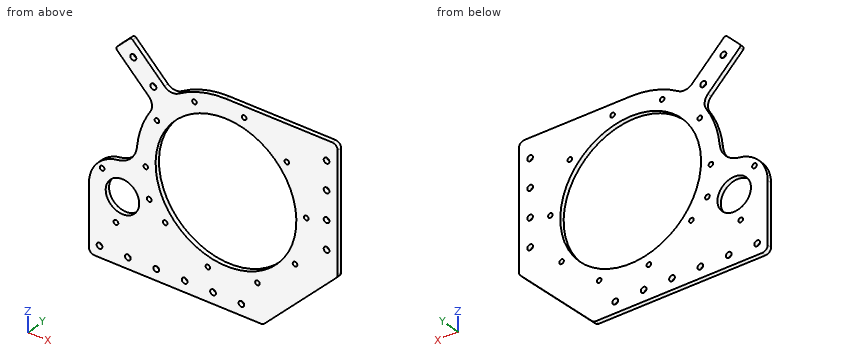
```python
from build123d import *

# Parameters (mm, degrees)
SKETCH_1_R               = 80
SKETCH_1_R_2             = 63
EXTRUDE_1_DEPTH          = 4
EXTRUDE_START            = -4
EXTRUDE_2_DEPTH          = 4
SKETCH_3_R               = 2.1
CUT_EXTRUDE_1_DEPTH      = 10
SKETCH_4_R               = 2.05
CUT_EXTRUDE_2_DEPTH      = 10
PATTERN_CIRCULAR_1_COUNT = 10
SKETCH_5_W               = 20
SKETCH_5_H               = 113.13708499
SKETCH_5_W_2             = 155.80242317
SKETCH_5_H_2             = 20
EXTRUDE_3_DEPTH          = 4
SKETCH_6_R               = 2.55
CUT_EXTRUDE_3_DEPTH      = 10
FILLET_1_R               = 20
SKETCH_7_R               = 15
CUT_EXTRUDE_4_DEPTH      = 10
FILLET_2_R               = 5
SKETCH_8_W               = 256.678769512
SKETCH_8_H               = 176.797047192
CUT_EXTRUDE_5_DEPTH      = 290
EXTRUDE_4_DEPTH          = 4
FILLET_3_R               = 10
FILLET_4_R               = 2
CUT_EXTRUDE_6_DEPTH      = 10


with BuildPart() as part:
    # 草图1 → 凸台-拉伸1 (new body)
    # profile 1 of 5: a face of its own
    with BuildSketch(Plane(origin=(0, 0, 0), x_dir=(1, 0, 0), z_dir=(0, 1, 0))):
        with BuildLine():
            ThreePointArc((0, -80), (-56.568542608, -56.568542382), (-80, 3.2e-07))
            Line((-80, 3.2e-07), (-80, -80))
            Line((-80, -80), (0, -80))
        make_face()
    # profile 2 of 5: a face of its own
    with BuildSketch(Plane(origin=(0, 0, 0), x_dir=(1, 0, 0), z_dir=(0, 1, 0))):
        Circle(SKETCH_1_R)
        with Locations(Location((0, 0, 0), (0, 0, 270))):
            Circle(SKETCH_1_R_2, mode=Mode.SUBTRACT)
    # profile 3 of 5: a face of its own
    with BuildSketch(Plane(origin=(0, 0, 0), x_dir=(1, 0, 0), z_dir=(0, 1, 0))):
        with BuildLine():
            ThreePointArc((-80, 3.2e-07), (-73.91036254, 30.614674737), (-56.568542495, 56.568542495))
            Line((-56.568542495, 56.568542495), (-80, 33.13708499))
            Line((-80, 33.13708499), (-80, 3.2e-07))
        make_face()
    # profile 4 of 5: a face of its own
    with BuildSketch(Plane(origin=(0, 0, 0), x_dir=(1, 0, 0), z_dir=(0, 1, 0))):
        with BuildLine():
            Line((0, 80), (-33.13708499, 80))
            Line((-33.13708499, 80), (-56.568542495, 56.568542495))
            ThreePointArc((-56.568542495, 56.568542495), (-30.614674589, 73.910362601), (0, 80))
        make_face()
    # profile 5 of 5: a face of its own
    with BuildSketch(Plane(origin=(0, 0, 0), x_dir=(1, 0, 0), z_dir=(0, 1, 0))):
        with BuildLine():
            Line((80, 80), (0, 80))
            ThreePointArc((0, 80), (56.568542495, 56.568542495), (80, 0))
            Line((80, 0), (80, 80))
        make_face()
    extrude(amount=EXTRUDE_1_DEPTH)


with BuildPart() as body_2:
    # 草图2 → 凸台-拉伸2 (new body)
    with BuildSketch(Plane(origin=(0, 4, 0), x_dir=(1, 0, 0), z_dir=(0, 1, 0)).offset(EXTRUDE_START)):
        with BuildLine():
            Line((122.66533818, 80), (80, 80))
            Line((80, 80), (80, 10))
            Line((80, 10), (92.66533818, 10))
            ThreePointArc((92.66533818, 10), (113.878541616, 18.786796564), (122.66533818, 40))
            Line((122.66533818, 40), (122.66533818, 80))
        make_face()
    extrude(amount=EXTRUDE_2_DEPTH)


with BuildPart() as part_1:
    add(part.part)

    # Combine 5: union body 2
    add(body_2.part)

    # 草图3 → 切除-拉伸1 (cut)
    with BuildSketch(Plane(origin=(0, 4, 0), x_dir=(1, 0, 0), z_dir=(0, 1, 0))):
        with Locations(Location((98.488743184, 64.31230047, 0), (0, 0, 270))):
            Circle(SKETCH_3_R)
        with Locations(Location((110.808705509, 22.800633094, 0), (0, 0, 270))):
            Circle(SKETCH_3_R)
        with Locations(Location((68.698565846, 32.887066435, 0), (0, 0, 270))):
            Circle(SKETCH_3_R)
    extrude(amount=-CUT_EXTRUDE_1_DEPTH, mode=Mode.SUBTRACT)

    # 草图4 → 切除-拉伸2 (cut)
    with BuildSketch(Plane(origin=(0, 4, 0), x_dir=(1, 0, 0), z_dir=(0, 1, 0))):
        with Locations(Location((-71.825637732, -6.283929052, 0), (0, 0, 270))):
            Circle(SKETCH_4_R)
    cut_extrude_2 = extrude(amount=-CUT_EXTRUDE_2_DEPTH, mode=Mode.SUBTRACT)

    # 阵列(圆周)1: 切除-拉伸2 ×10 about axis
    pattern_circular_1_axis = Axis((0, 0, 0), (0, 1, 0))
    for i in range(1, PATTERN_CIRCULAR_1_COUNT):
        add(cut_extrude_2.rotate(pattern_circular_1_axis, i * 360 / PATTERN_CIRCULAR_1_COUNT), mode=Mode.SUBTRACT)

    # 草图5 → 凸台-拉伸3 (add)
    with BuildSketch(Plane(origin=(0, 4, 0), x_dir=(1, 0, 0), z_dir=(0, 1, 0))):
        with Locations((-90, -23.431457505)):
            Rectangle(SKETCH_5_W, SKETCH_5_H)
        Polygon((-33.13708499, 80), (-33.13708499, 100), (-100, 33.13708499), (-80, 33.13708499), align=None)
        with Locations((44.764126595, 90)):
            Rectangle(SKETCH_5_W_2, SKETCH_5_H_2)
    extrude(amount=-EXTRUDE_3_DEPTH)

    # 草图6 → 切除-拉伸3 (cut)
    with BuildSketch(Plane(origin=(0, 4, 0), x_dir=(1, 0, 0), z_dir=(0, 1, 0))):
        with Locations(Location((-13.8, 90, 0), (0, 0, 270))):
            Circle(SKETCH_6_R)
        with Locations(Location((11.6, 90, 0), (0, 0, 270))):
            Circle(SKETCH_6_R)
        with Locations(Location((37, 90, 0), (0, 0, 270))):
            Circle(SKETCH_6_R)
        with Locations(Location((62.4, 90, 0), (0, 0, 270))):
            Circle(SKETCH_6_R)
        with Locations(Location((87.8, 90, 0), (0, 0, 270))):
            Circle(SKETCH_6_R)
        with Locations(Location((113.2, 90, 0), (0, 0, 270))):
            Circle(SKETCH_6_R)
        with Locations(Location((-90, 13.8, 0), (0, 0, 270))):
            Circle(SKETCH_6_R)
        with Locations(Location((-90, -11.6, 0), (0, 0, 270))):
            Circle(SKETCH_6_R)
        with Locations(Location((-90, -37, 0), (0, 0, 270))):
            Circle(SKETCH_6_R)
        with Locations(Location((-90, -62.4, 0), (0, 0, 270))):
            Circle(SKETCH_6_R)
    extrude(amount=-CUT_EXTRUDE_3_DEPTH, mode=Mode.SUBTRACT)

    # 圆角1
    fillet_1_edges = [part_1.edges().sort_by_distance(p)[0] for p in [
        (80, 2, -10),
    ]]
    fillet(fillet_1_edges, radius=FILLET_1_R)

    # 草图7 → 切除-拉伸4 (cut)
    with BuildSketch(Plane(origin=(0, 4, 0), x_dir=(1, 0, 0), z_dir=(0, 1, 0))):
        with Locations(Location((92.66533818, 40, 0), (0, 0, 270))):
            Circle(SKETCH_7_R)
    extrude(amount=-CUT_EXTRUDE_4_DEPTH, mode=Mode.SUBTRACT)

    # 圆角2
    fillet_2_edges = [part_1.edges().sort_by_distance(p)[0] for p in [
        (-100, 2, 80),
        (-100, 2, -33.13708499),
        (-33.13708499, 2, -100),
        (122.66533818, 2, -100),
    ]]
    fillet(fillet_2_edges, radius=FILLET_2_R)


with BuildPart() as body_2_2:
    # 镜向2: mirrored copy
    add(part_1.part.mirror(Plane(origin=(132.66533818, 0, 0), x_dir=(0, 0, 1), z_dir=(1, 0, 0))))

    # 草图9 → 凸台-拉伸4 (add)
    with BuildSketch(Plane(origin=(0, 4, 0), x_dir=(1, 0, 0), z_dir=(0, 1, 0))):
        with BuildLine():
            Line((166.335726994, -84.852813742), (180.477862617, -98.994949366))
            Line((180.477862617, -98.994949366), (216.27688337, -63.195928613))
            ThreePointArc((216.27688337, -63.195928613), (208.762133865, -56.568542495), (202.134747746, -49.05379299))
            Line((202.134747746, -49.05379299), (166.335726994, -84.852813742))
        make_face()
    extrude(amount=-EXTRUDE_4_DEPTH)

    # 圆角3
    fillet_3_edges = [body_2_2.edges().sort_by_distance(p)[0] for p in [
        (202.134747746, 2, 49.05379299),
        (216.27688337, 2, 63.195928613),
    ]]
    fillet(fillet_3_edges, radius=FILLET_3_R)

    # 圆角4
    fillet_4_edges = [body_2_2.edges().sort_by_distance(p)[0] for p in [
        (166.335726994, 2, 84.852813742),
        (180.477862617, 2, 98.994949366),
    ]]
    fillet(fillet_4_edges, radius=FILLET_4_R)

    # 草图10 → 切除-拉伸6 (cut)
    with BuildSketch(Plane(origin=(0, 4, 0), x_dir=(1, 0, 0), z_dir=(0, 1, 0))):
        with BuildLine():
            ThreePointArc((202.221396139, -63.109280221), (198.473730199, -63.109280221), (198.473730199, -66.856946161))
            Line((198.473730199, -66.856946161), (202.221396139, -63.109280221))
        make_face()
        with BuildLine():
            Line((202.221396139, -63.109280221), (198.473730199, -66.856946161))
            ThreePointArc((198.473730199, -66.856946161), (201.361674265, -67.431393952), (202.997563169, -64.983113191))
            ThreePointArc((202.997563169, -64.983113191), (202.79584393, -63.969002095), (202.221396139, -63.109280221))
        make_face()
        with BuildLine():
            ThreePointArc((184.260883897, -81.069792463), (180.513217957, -81.069792463), (180.513217957, -84.817458403))
            Line((180.513217957, -84.817458403), (184.260883897, -81.069792463))
        make_face()
        with BuildLine():
            Line((184.260883897, -81.069792463), (180.513217957, -84.817458403))
            ThreePointArc((180.513217957, -84.817458403), (183.401162022, -85.391906194), (185.037050927, -82.943625433))
            ThreePointArc((185.037050927, -82.943625433), (184.835331688, -81.929514337), (184.260883897, -81.069792463))
        make_face()
    extrude(amount=-CUT_EXTRUDE_6_DEPTH, mode=Mode.SUBTRACT)


with BuildPart() as part_2:
    add(part_1.part)

    # 草图8 → 切除-拉伸5 (cut)
    with BuildSketch(Plane(origin=(132.66533818, 0, 0), x_dir=(0, 0, -1), z_dir=(1, 0, 0))):
        with Locations((25.923800224, 29.064395705)):
            Rectangle(SKETCH_8_W, SKETCH_8_H)
    extrude(amount=-CUT_EXTRUDE_5_DEPTH, mode=Mode.SUBTRACT)


solid = body_2_2.part
```
Verification items for the finished model (mm, model axes). Give positions to 0.01 mm unless a question says otherwise; leave off trailing zeros. Loops run counter-clockwise (first coordinate to the right, second up) from the corner with the lowest first, then second, coordinate; pieces in that order, holes last.
1. Section check C-C, the plane z = -90. Enter the section's corners in (x, y).
2. Section check B-B, the plane z = -13.8. Enter the section's corners in (x, y).
3. Thickness scan on line 1 (X direction, y = 1, z = -53); line 2 (Z direction, x = 256, y = 2.7); line 3 (Z direction, x = 278, y = 2.65). Record the ranges inside material, lowest first.
4. Section check D-D, the plane y = 1.45. Count the separate pieces of the cut face and the enclosed holes in it, then the cut area to 3 significant figures.
5. Section check A-A, the plane x = 273.5. Enter the section's corners in (y, z), then the cut area to 3 significant figures.
6. Go/stop test with flat-tipped pins: pin 1 Ø1.5 at (y, z) = (3.5, -72) entering from +X; pin 2 Ø2 at (y, z) = (2.5, 62) entering from -X; pin 3 Ø1.5 at (x, y) = (228.5, 3) entering from +Z. Record where each tip stops, or that it passes through.
Geometry says:
1. outline: (142.67, 0) - (149.58, 0) - (149.58, 4) - (142.67, 4) - close; (154.68, 0) - (174.98, 0) - (174.98, 4) - (154.68, 4) - close; (180.08, 0) - (200.38, 0) - (200.38, 4) - (180.08, 4) - close; (205.48, 0) - (225.78, 0) - (225.78, 4) - (205.48, 4) - close; (230.88, 0) - (251.18, 0) - (251.18, 4) - (230.88, 4) - close; (256.28, 0) - (276.58, 0) - (276.58, 4) - (256.28, 4) - close; (281.68, 0) - (308.47, 0) - (308.47, 4) - (281.68, 4) - close
2. outline: (158.05, 0) - (203.86, 0) - (203.86, 4) - (158.05, 4) - close; (326.8, 0) - (352.78, 0) - (352.78, 4) - (326.8, 4) - close; (357.88, 0) - (365.33, 0) - (365.33, 4) - (357.88, 4) - close
3. line 1: x = 142.67 to 165.18, 180.15 to 231.27, 299.39 to 345.47
3. line 2: z = -100 to -91.16, -88.84 to -62.31, 62.31 to 79.45
3. line 3: z = -100 to -92.29, -87.71 to -61.71, 61.71 to 80
4. separate pieces: 1
4. enclosed holes: 27
4. area: 19,900 mm2
5. outline: (0, -100) - (4, -100) - (4, -62.47) - (0, -62.47) - close; (0, 62.47) - (4, 62.47) - (4, 80) - (0, 80) - close
5. area: 220 mm2
6. pin 1: stops at x = 327.22
6. pin 2: stops at x = 188.19
6. pin 3: stops at z = 71.4
